Build history of the part. All positions in model axes, mm. A direction names the side the tool comes from. Round coordinates to 2 decimals unless told otherwise and drop trailing zeros. Write each loop counter-clockwise with the first axis right and the second up, starting at its lowest first coordinate (ties: lowest second). Pieces come first, ordered by that corner, then holes. Notation, with made-up numbers: M 60,82.25 L 79,82.25 A20 ccw 79,88.25 Z; hole C 5.25,-38 d7. An arc over 180 degrees is marked long. Use a Markdown table: item, result.
from build123d import *

# Parameters (mm, degrees)
SKETCH_1_W          = 40
SKETCH_1_H          = 20
EXTRUDE_1_DEPTH     = 6
SKETCH_2_W          = 40
SKETCH_2_H          = 32.5
EXTRUDE_2_DEPTH     = 35
CUT_EXTRUDE_1_DEPTH = 13
CUT_EXTRUDE_2_DEPTH = 2
SKETCH_6_W          = 40
SKETCH_6_H          = 41
CUT_EXTRUDE_3_DEPTH = 5
SKETCH_8_R          = 1.7
SKETCH_8_R_2        = 1.4
CUT_EXTRUDE_4_DEPTH = 49.79805324
CUT_EXTRUDE_5_REACH = 48.165
SKETCH_9_W          = 40
SKETCH_9_H          = 3
CHAMFER_1_SIZE2     = 6
CHAMFER_1_SIZE      = 0.8
CUT_EXTRUDE_6_REACH = 49.173
SKETCH_11_W         = 0.4
SKETCH_11_H         = 41


with BuildPart() as part:
    # Эскиз1 → Бобышка-Вытянуть1 (new body)
    with BuildSketch(Plane.XY):
        Rectangle(SKETCH_1_W, SKETCH_1_H)
    extrude(amount=EXTRUDE_1_DEPTH)

    # Эскиз2 → Бобышка-Вытянуть2 (add)
    with BuildSketch(Plane(origin=(0, 0, 0), x_dir=(-1, 0, 0), z_dir=(0, 0, -1))):
        with Locations((0, 6.25)):
            Rectangle(SKETCH_2_W, SKETCH_2_H)
    extrude(amount=EXTRUDE_2_DEPTH)

    # Эскиз3 → Вырез-Вытянуть1 (cut)
    with BuildSketch(Plane.XZ.offset(10)):
        Polygon((-7, 6), (-7, -1), (-9, -1), (-9, -23), (-6.5, -26), (-6.5, -33), (-4.5, -33), (-4.5, -35), (4.5, -35), (4.5, -33), (6.5, -33), (6.5, -26), (9, -23), (9, -1), (7, -1), (7, 6), align=None)
    extrude(amount=-CUT_EXTRUDE_1_DEPTH, mode=Mode.SUBTRACT)

    # Эскиз5 → Вырез-Вытянуть2 (cut)
    with BuildSketch(Plane.XZ.offset(-3)):
        Polygon((-9, -1), (9, -1), (9, -23), (6.5, -26), (6.5, -33), (-6.5, -33), (-6.5, -26), (-9, -23), align=None)
    extrude(amount=-CUT_EXTRUDE_2_DEPTH, mode=Mode.SUBTRACT)

    # Эскиз6 → Вырез-Вытянуть3 (cut)
    with BuildSketch(Plane.XZ.offset(10)):
        with Locations((0, -14.5)):
            Rectangle(SKETCH_6_W, SKETCH_6_H)
    extrude(amount=-CUT_EXTRUDE_3_DEPTH, mode=Mode.SUBTRACT)

    # Эскиз8 → Вырез-Вытянуть4 (cut, through all)
    with BuildSketch(Plane.XZ.offset(5)):
        with Locations((12, -26)):
            Circle(SKETCH_8_R)
        with Locations((14.5, -6)):
            Circle(SKETCH_8_R_2)
        with Locations(Location((-12, -26, 0), (0, 0, 180))):
            Circle(SKETCH_8_R)
        with Locations(Location((-14.5, -6, 0), (0, 0, 180))):
            Circle(SKETCH_8_R_2)
    extrude(amount=-CUT_EXTRUDE_4_DEPTH, mode=Mode.SUBTRACT)

    # Вырез-Вытянуть5: up to this face of the body (flat: up to its plane)
    cut_extrude_5_end = Plane(part.part.faces().sort_by_distance((0, 9.432879377, -35))[0])
    # Эскиз9 → Вырез-Вытянуть5 (cut, up to the picked face)
    with BuildSketch(Plane.XY, mode=Mode.PRIVATE) as cut_extrude_5_sk1:
        with Locations((0, 21)):
            Rectangle(SKETCH_9_W, SKETCH_9_H)
    cut_extrude_5_tool1 = split(extrude(cut_extrude_5_sk1.sketch, amount=-CUT_EXTRUDE_5_REACH, mode=Mode.PRIVATE), bisect_by=cut_extrude_5_end, keep=Keep.BOTH, mode=Mode.PRIVATE)
    add(cut_extrude_5_tool1.solids().sort_by(Axis((0, 21, 0), (0, 0, -1)))[0], mode=Mode.SUBTRACT)

    # Фаска1
    chamfer_1_edges = [part.edges().sort_by_distance(p)[0] for p in [
        (0, 10, 6),
    ]]
    chamfer_1_side = [part.faces().sort_by_distance(p)[0] for p in [
        (0, 9.984, 6),
    ]]
    chamfer(chamfer_1_edges, length=CHAMFER_1_SIZE - 0.0001, length2=CHAMFER_1_SIZE2 - 0.0001, reference=chamfer_1_side[0])  # a hair under: the kernel refuses the full size

    # Вырез-Вытянуть6: up to this face of the body (flat: up to its plane)
    cut_extrude_6_end = Plane(part.part.faces().sort_by_distance((13.916834893, -5, -14.890204003))[0])
    # Эскиз11 → Вырез-Вытянуть6 (cut, up to the picked face)
    with BuildSketch(Plane(origin=(0, 19.5, 0), x_dir=(1, 0, 0), z_dir=(0, 1, 0)), mode=Mode.PRIVATE) as cut_extrude_6_sk1:
        with Locations((-19.8, 14.5)):
            Rectangle(SKETCH_11_W, SKETCH_11_H)
    cut_extrude_6_tool1 = split(extrude(cut_extrude_6_sk1.sketch, amount=-CUT_EXTRUDE_6_REACH, mode=Mode.PRIVATE), bisect_by=cut_extrude_6_end, keep=Keep.BOTH, mode=Mode.PRIVATE)
    # Эскиз11 → Вырез-Вытянуть6 (cut, up to the picked face)
    with BuildSketch(Plane(origin=(0, 19.5, 0), x_dir=(1, 0, 0), z_dir=(0, 1, 0)), mode=Mode.PRIVATE) as cut_extrude_6_sk2:
        with Locations((19.8, 14.5)):
            Rectangle(SKETCH_11_W, SKETCH_11_H)
    cut_extrude_6_tool2 = split(extrude(cut_extrude_6_sk2.sketch, amount=-CUT_EXTRUDE_6_REACH, mode=Mode.PRIVATE), bisect_by=cut_extrude_6_end, keep=Keep.BOTH, mode=Mode.PRIVATE)
    add(cut_extrude_6_tool1.solids().sort_by(Axis((-19.8, 19.5, -14.5), (0, -1, 0)))[0], mode=Mode.SUBTRACT)
    add(cut_extrude_6_tool2.solids().sort_by(Axis((19.8, 19.5, -14.5), (0, -1, 0)))[0], mode=Mode.SUBTRACT)


solid = part.part
Q1. Cut at C-C on z = -32. Give the cut face in (x, y), and give its area (3 significant figures).
Response values:
| item | result |
|---|---|
| outline | M -19.6,-5 L -6.5,-5 L -6.5,5 L 6.5,5 L 6.5,-5 L 19.6,-5 L 19.6,19.5 L -19.6,19.5 Z |
| area | 830 mm2 |
Q2. Cut at B-B on y = 1. Give the cut face in (x, z), and give its area (3 significant figures).
Response values:
| item | result |
|---|---|
| outline | M -19.6,-35 L -4.5,-35 L -4.5,-33 L -6.5,-33 L -6.5,-26 L -9,-23 L -9,-1 L -7,-1 L -7,6 L -19.6,6 Z; M 4.5,-35 L 19.6,-35 L 19.6,6 L 7,6 L 7,-1 L 9,-1 L 9,-23 L 6.5,-26 L 6.5,-33 L 4.5,-33 Z; hole C -14.5,-6 d2.8; hole C -12,-26 d3.4; hole C 12,-26 d3.4; hole C 14.5,-6 d2.8 |
| area | 927 mm2 |
Q3. Cut at D-D on y = 7.5. Give the cut face in (x, z), and give its area (3 significant figures).
Response values:
| item | result |
|---|---|
| outline | M -19.6,-35 L 19.6,-35 L 19.6,6 L -19.6,6 Z; hole C -14.5,-6 d2.8; hole C -12,-26 d3.4; hole C 12,-26 d3.4; hole C 14.5,-6 d2.8 |
| area | 1,580 mm2 |
Q4. Drop flat-ended pins along their axis: P1, Ø5.5, axis at x = 1.5, z = 4, coming from the -Y side; P2, Ø1, axis at x = -2.5, z = -5.5, coming from the -Y side; P3, Ø5, axis at x = 3, y = -1.5, coming from the +Z side. Give the stop position or say it passes through.
Response values:
| item | result |
|---|---|
| P1 | stops at y = 3 |
| P2 | stops at y = 5 |
| P3 | stops at z = -33 |
Q5. Drill centre lines: L1, parallel to X at y = 0.75, z = -9; L2, parallel to Z at x = 12, y = 11.5; L3, parallel to Z at x = -12, y = 3.5. Where is each one in solid material? Low to high.
Response values:
| item | result |
|---|---|
| L1 | x = -19.6 to -9, 9 to 19.6 |
| L2 | z = -35 to -27.7, -24.3 to 0 |
| L3 | z = -35 to -27.7, -24.3 to 6 |
Q6. Two-plate mould, pull along Z, no slides. Class faces 4 (the flat face through (14, -5, -14)), 5 (the flat face through (0, 15, 0)), 6 (the cylindrical face through (12.914, 7.078, -24.567)): +Z half, -Z half, draft (parallel to the pull), parting line (faces both ways), or undercut.
Response values:
| item | result |
|---|---|
| face 4 | draft |
| face 5 | +Z half |
| face 6 | undercut |
Q7. Which spindle directions (+Z, -Z, +X, -X, +Y, -Y) get a long thin tool onto all of the face, cutting with end or side? Do faces 1 (the flat face through (0, 3, 3)), 2 (the flat face through (-9, 0, -12)), 3 (the flat face through (0, 4, 6)). Say none if no direction does.
Response values:
| item | result |
|---|---|
| face 1 | +Z, -Y |
| face 2 | -Y |
| face 3 | +Z, +X, -X, +Y, -Y |
